```python
from build123d import *

# Parameters (mm, degrees)
F1_DEPTH = 25
F2_DEPTH = 40
F3_R     = 12.5
F4_DEPTH = 40.001
F5_R     = 25
F6_DEPTH = 15
F7_R     = 10
F9_DEPTH = 10
F10_R    = 10


with BuildPart() as f1:
    # F0 (on Top) → F1 (new body)
    with BuildSketch(Plane.XY):
        with BuildLine():
            ThreePointArc((-10, 48.989795), (31.622777, 38.729833), (50, 0))
            Line((50, 0), (50, 165))
            Line((50, 165), (-10, 165))
            Line((-10, 165), (-10, 48.989795))
        make_face()
    extrude(amount=-F1_DEPTH)

    # F0 (on Top) → F2 (join)
    with BuildSketch(Plane.XY):
        with BuildLine():
            Line((-10, 0), (50, 0))
            ThreePointArc((50, 0), (31.622777, 38.729833), (-10, 48.989795))
            Line((-10, 48.989795), (-10, 0))
        make_face()
        with BuildLine():
            ThreePointArc((-10, 48.989795), (-31.622777, -38.729833), (50, 0))
            Line((50, 0), (-10, 0))
            Line((-10, 0), (-10, 48.989795))
        make_face()
    extrude(amount=-F2_DEPTH)

    # F3 (on face) → F4 (cut, through all)
    with BuildSketch(Plane(origin=(0, 0, -40), x_dir=(1, 0, 0), z_dir=(0, 0, -1))):
        Circle(F3_R)
    extrude(amount=-F4_DEPTH, mode=Mode.SUBTRACT)

    # F5 (on face) → F6 (cut)
    with BuildSketch(Plane(origin=(0, 0, -40), x_dir=(1, 0, 0), z_dir=(0, 0, -1))):
        Circle(F5_R)
    extrude(amount=-F6_DEPTH, mode=Mode.SUBTRACT)

    # F7
    f7_edges = [f1.edges().sort_by_distance(p)[0] for p in [
        (-10, 165, -12.5),
        (50, 165, -12.5),
    ]]
    fillet(f7_edges, radius=F7_R)

    # F8 (on face) → F9 (cut)
    with BuildSketch(Plane(origin=(0, 0, -25), x_dir=(1, 0, 0), z_dir=(0, 0, -1))):
        with BuildLine():
            Line((0, -155), (40, -155))
            Line((40, -155), (40, -44.72136))
            ThreePointArc((40, -44.72136), (21.409325, -56.050342), (0, -60))
            Line((0, -60), (0, -155))
        make_face()
    extrude(amount=-F9_DEPTH, mode=Mode.SUBTRACT)

    # F10
    f10_edges = [f1.edges().sort_by_distance(p)[0] for p in [
        (0, 155, -20),
        (40, 155, -20),
    ]]
    fillet(f10_edges, radius=F10_R)


solid = f1.part
```
Check sheet for the modelled part. Datum: model origin and axes. Units: mm. A direction names the side the tool comes from. Round coordinates to 2 decimals unless told otherwise and drop trailing zeros. Order: outer loops, then holes, each group sorted by start corner. A loop starts at its lowest first (then second) coordinate and runs counter-clockwise, first axis right, second up.
1) Section check C-C (x = 2). Record the boundary of the cut face in (y, z), and give its area (3 significant figures).
2) Section check A-A (z = -7). Record the boundary of the cut face in (x, y), and give its area (3 significant figures).
3) Mould release check, pull along X, two halves, no side actions. Record for faces 1 (the flat face through (-10, 103, -12)), 2 (the flat face through (50, 76, -12)), 3 (the flat face through (-11.5, -5.9, -25)), 4 (the flat face through (20, 155, -20)): +X half, -X half, draft (parallel to the pull), parting line (faces both ways), or undercut.
4) Go/stop test with flat-tipped pins: pin 1 Ø3 at (y, z) = (100.5, -22) entering from -X; pin 2 Ø2 at (x, y) = (34, 59) entering from +Z; pin 3 Ø3 at (x, z) = (20.5, -19.5) entering from -Y; pin 4 Ø10 at (x, z) = (-38.5, -35) entering from -Y. Record where each tip stops, or that it passes through.
5) Section check B-B (y = 109). Record the boundary of the cut face in (x, z).
6) Scan lines: line 1 (Y direction, x = 0, z = -6); line 2 (X direction, y = 0, z = -14.25); line 3 (X direction, y = 129.5, z = -10.5). Record each from-to range of solid material in increasing order.
7) Tool access check on faces 5 (the flat face through (42, 95, -25)), 6 (the flat face through (0, 102, -20)), 7 (the cylindrical face through (-6.99, 162.15, -12.68)). Record the directions out of +Z, -Z, +X, -X, +Y, -Y that give a thin tool (end or side, any length) a straight path to the whole face; none if there is none.
8) Section check D-D (x = 28). Record the boundary of the cut face in (y, z), and give its area (3 significant figures).
Result:
1. outline: (-49.96, -40) - (-24.92, -40) - (-24.92, -25) - (-12.34, -25) - (-12.34, 0) - (-49.96, 0) - close; (12.34, -25) - (24.92, -25) - (24.92, -40) - (49.96, -40) - (49.96, -25) - (59.97, -25) - (59.97, -15) - (151, -15) - (151, -25) - (165, -25) - (165, 0) - (12.34, 0) - close
1. area: 4,600 mm2
2. outline: (-10, 48.99) arc R50 ccw (long way) to (50, 0) - (50, 155) arc R10 ccw to (40, 165) - (0, 165) arc R10 ccw to (-10, 155) - close; hole circle Ø25 at (0, 0)
2. area: 14,800 mm2
3. face 1: -X half
3. face 2: +X half
3. face 3: undercut
3. face 4: undercut
4. pin 1: stops at x = -10
4. pin 2: stops at z = 0
4. pin 3: stops at y = -46.25
4. pin 4: stops at y = -37.12
5. outline: (-10, -25) - (0, -25) - (0, -15) - (40, -15) - (40, -25) - (50, -25) - (50, 0) - (-10, 0) - close
6. line 1: y = -50 to -12.5, 12.5 to 165
6. line 2: x = -50 to -12.5, 12.5 to 50
6. line 3: x = -10 to 50
7. face 5: -Z, +X, +Y
7. face 6: -Z
7. face 7: +Z, -Z, -X, +Y
8. outline: (-41.42, -40) - (41.42, -40) - (41.42, -25) - (53.07, -25) - (53.07, -15) - (155, -15) - (155, -25) - (165, -25) - (165, 0) - (-41.42, 0) - close
8. area: 5,380 mm2
